```python
from build123d import *

# Parameters (mm, degrees)
SKETCH1_W           = 30
SKETCH1_H           = 16
BOSS_EXTRUDE1_DEPTH = 2
SKETCH4_W           = 5
SKETCH4_H           = 4
BOSS_EXTRUDE2_DEPTH = 0.5
CIRPATTERN1_COUNT   = 4


with BuildPart() as part:
    # Sketch1 → Boss-Extrude1 (new body)
    with BuildSketch(Plane(origin=(0, 0, 0), x_dir=(1, 0, 0), z_dir=(0, 1, 0))):
        Rectangle(SKETCH1_W, SKETCH1_H)
    extrude(amount=BOSS_EXTRUDE1_DEPTH)

    # Sketch4 → Boss-Extrude2 (add)
    with BuildSketch(Plane(origin=(-2.349067885, 3.959105139, 2.349067885), x_dir=(0.7071067811865479, 0, 0.7071067811865471), z_dir=(0.4545194776720462, -0.7660444431189748, -0.4545194776720467))):
        with Locations((0, 1.047826544)):
            Rectangle(SKETCH4_W, SKETCH4_H)
    boss_extrude2 = extrude(amount=BOSS_EXTRUDE2_DEPTH)

    # CirPattern1: Boss-Extrude2 ×4 about axis
    cirpattern1_axis = Axis((0, 0, 0), (0, 1, 0))
    for i in range(1, CIRPATTERN1_COUNT):
        add(boss_extrude2.rotate(cirpattern1_axis, i * 360 / CIRPATTERN1_COUNT))


solid = part.part
```
Input: part model. Units: mm. Frame: model coordinates. A direction names the side the tool comes from. Round coordinates to 2 decimals unless told otherwise and drop trailing zeros. Write each loop counter-clockwise with the first axis right and the second up, starting at its lowest first coordinate (ties: lowest second). Pieces come first, ordered by that corner, then holes. Notation, with made-up numbers: M 13,23 L 32,23 A30 ccw 32,53 Z; hole C 69,-29 d2. An arc over 180 degrees is marked long. Write each question's results on one line, items separated by ' | '.
Q1. Section query B-B (x = 0.75). Return loops of the section in (y, z).
Results:
outline: M 0,-8 L 2,-8 L 2,8 L 0,8 Z; M 3.11,-4.29 L 3.76,-4.29 L 4.57,-2.92 L 4.19,-2.46 Z; M 3.11,4.29 L 4.19,2.46 L 4.57,2.92 L 3.76,4.29 Z
Q2. Draft query along Z for faces 6 (the face through (-2.957, 3.268, 2.907)), 7 (the face through (-2.907, 3.268, -2.957)), 8 (the face through (1.746, 4.382, -1.697)). Return one class per face: released by +Z, released by -Z, zero draft, split by the parting line, or undercut.
Results:
face 6: released by +Z | face 7: released by -Z | face 8: undercut
Q3. Section query D-D (x = -6.25). Return loops of the section in (y, z).
Results:
outline: M 0,-8 L 2,-8 L 2,8 L 0,8 Z
Q4. Section query C-C (z = -4). Return loops of the section in (x, y), and give its area (3 significant figures).
Results:
outline: M -15,0 L 15,0 L 15,2 L 4,2 L 0.46,4.1 L 0.46,3.45 L 2.9,2 L -2.9,2 L -0.46,3.45 L -0.46,4.1 L -4,2 L -15,2 Z | area: 63.9 mm^2
Q5. Access query for faces 1 (the face through (4.557, 3.115, -1.022)), 2 (the face through (1.697, 4.382, 1.746)), 3 (the face through (2.516, 3.079, 2.566)), 4 (the face through (1.022, 3.115, 4.557)), 5 (the face through (1.022, 3.115, -4.557)). Directions: +Z, -Z, +X, -X, +Y, -Y. A direction counts if a zero-diameter tool reaches every point of the face in a straight line with its end or side. Return the directions, or none.
Results:
face 1: +X, +Y | face 2: +Y | face 3: none | face 4: +Z, +Y | face 5: -Z, +Y
Q6. Section query A-A (y = 3.4). Return loops of the section in (x, z).
Results:
outline: M -4.59,-1.05 L -1.05,-4.59 L -0.5,-4.04 L -4.04,-0.5 Z; M -4.59,1.05 L -4.04,0.5 L -0.5,4.04 L -1.05,4.59 Z; M 0.5,-4.04 L 1.05,-4.59 L 4.59,-1.05 L 4.04,-0.5 Z; M 0.5,4.04 L 4.04,0.5 L 4.59,1.05 L 1.05,4.59 Z
Q7. Line query: line 1 along Y through (x, z) = (-3.75, -6.5); line 2 along X through (y, z) = (2.25, 3.25); line 3 along X through (y, z) = (3.95, -3.5). Output: solid intervals per line, ascending.
Results:
line 1: y = 0 to 2 | line 2: x = -4.33 to -3.23, 3.23 to 4.33 | line 3: x = -1.21 to -0.11, 0.11 to 1.21
